Verification items for the finished model (mm, model axes). Face numbers are marked on the shaded views. A direction names the side the tool comes from. Round coordinates to 2 decimals unless told otherwise and drop trailing zeros. Write each loop counter-clockwise with the first axis right and the second up, starting at its lowest first coordinate (ties: lowest second). Pieces come first, ordered by that corner, then holes.
from build123d import *

# Parameters (mm, degrees)
SKETCH_1_R           = 7.505
SKETCH_1_R_2         = 2.505
EXTRUDE_1_DEPTH      = 10
EXTRUDE_3_DEPTH      = 18.25
EXTRUDE_3_DEPTH_BACK = 7
SKETCH_7_W           = 8
SKETCH_7_H           = 10
SKETCH_9_W           = 8
SKETCH_9_H           = 3.5
CUT_EXTRUDE_1_DEPTH  = 18.25
SKETCH_10_R          = 7.505
SKETCH_10_R_2        = 2.505
EXTRUDE_4_DEPTH      = 10
SKETCH_11_R          = 2.505
CUT_EXTRUDE_2_DEPTH  = 10


with BuildPart() as part:
    # 草圖1 → 伸長-薄件1 (new body)
    with BuildSketch(Plane(origin=(0, 0, 0), x_dir=(1, 0, 0), z_dir=(0, 1, 0))):
        Circle(SKETCH_1_R)
        Circle(SKETCH_1_R_2, mode=Mode.SUBTRACT)
    extrude(amount=EXTRUDE_1_DEPTH)

    # 草圖7 → 填料-伸長3 (add, two sides: drawn at the far end of the back side and taken through both)
    with BuildSketch(Plane.XY.offset(13).offset(-EXTRUDE_3_DEPTH_BACK)):
        with Locations((0, 5)):
            Rectangle(SKETCH_7_W, SKETCH_7_H)
    extrude(amount=EXTRUDE_3_DEPTH + EXTRUDE_3_DEPTH_BACK)

    # 草圖9 → 除料-伸長1 (cut)
    with BuildSketch(Plane(origin=(0, 10, 0), x_dir=(1, 0, 0), z_dir=(0, 1, 0))):
        with Locations((0, -29.5)):
            Rectangle(SKETCH_9_W, SKETCH_9_H)
    extrude(amount=-CUT_EXTRUDE_1_DEPTH, mode=Mode.SUBTRACT)

    # 草圖10 → 伸長-薄件4 (add)
    with BuildSketch(Plane(origin=(0, 10, 0), x_dir=(1, 0, 0), z_dir=(0, 1, 0))):
        with Locations((0, -27.75)):
            Circle(SKETCH_10_R)
        with Locations((0, -27.75)):
            Circle(SKETCH_10_R_2, mode=Mode.SUBTRACT)
    extrude(amount=-EXTRUDE_4_DEPTH)

    # 草圖11 → 除料-伸長2 (cut)
    with BuildSketch(Plane(origin=(0, 10, 0), x_dir=(1, 0, 0), z_dir=(0, 1, 0))):
        with Locations(Location((0, -27.75, 0), (0, 0, 270))):
            Circle(SKETCH_11_R)
    extrude(amount=-CUT_EXTRUDE_2_DEPTH, mode=Mode.SUBTRACT)


solid = part.part
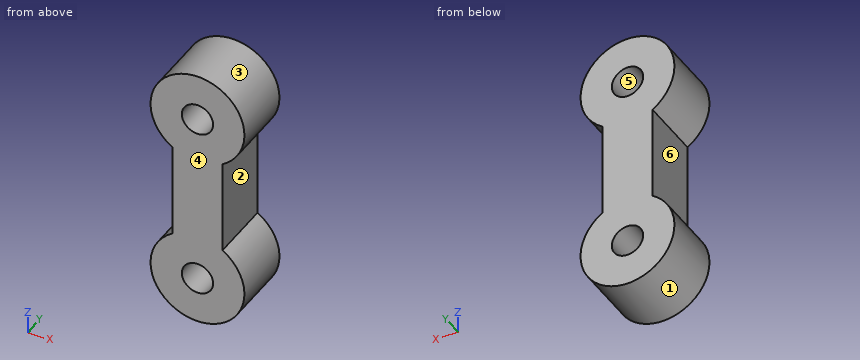
Q1. Depth check by flat-ended pin: P1, Ø5, axis at y = 5.5, z = 15.5, coming from the -X side; P2, Ø3, axis at x = 3, y = 4.5, coming from the -Z side; P3, Ø6, axis at y = 7.5, z = 9.5, coming from the +X side; P4, Ø4.5, axis at x = 0, z = 27.75, coming from the +Y side. Enter the tip coordinate at first touch or a pass-through.
Recorded:
P1: stops at x = -4
P2: stops at z = -7.35
P3: stops at x = 4
P4: passes through
Q2. Sectioned sample at B-B (z = 27.75). Enter the section's corners in (x, y) (3 decimals).
Recorded:
outline: (-7.505, 0) - (-2.505, 0) - (-2.505, 10) - (-7.505, 10) - close; (2.505, 0) - (7.505, 0) - (7.505, 10) - (2.505, 10) - close
Q3. Sectioned sample at D-D (y = 7). Enter the section's corners in (x, z) (3 decimals).
Recorded:
outline: (-4, 6.35) arc R7.505 ccw (long way) to (4, 6.35) - (4, 21.4) arc R7.505 ccw (long way) to (-4, 21.4) - close; hole circle Ø5.01 at (0, 0); hole circle Ø5.01 at (0, 27.75)
Q4. Release check for a two-part mould opening along X. For the marked faces 3, 4, 5 and 6 record: released by +X, released by -X, zero draft, split by the parting line, or undercut.
Recorded:
face 3: split by the parting line
face 4: zero draft
face 5: undercut
face 6: released by -X
Q5. Tool access check on the marked faces 1 and 2. Record the directions out of +Z, -Z, +X, -X, +Y, -Y that give a thin tool (end or side, any length) a straight path to the whole face; none if there is none.
Recorded:
face 1: +Y, -Y
face 2: +X, +Y, -Y
Q6. Material ranges on line 1 along Z through (x, y) = (0, 6.5) (3 decimals); line 2 along Z through (x, y) = (1.25, 3.25); line 3 along X through (y, z) = (2.5, 0) (3 decimals), recorded low to high.
Recorded:
line 1: z = -7.505 to -2.505, 2.505 to 25.245, 30.255 to 35.255
line 2: z = -7.4 to -2.17, 2.17 to 25.58, 29.92 to 35.15
line 3: x = -7.505 to -2.505, 2.505 to 7.505
Q7. Sectioned sample at A-A (x = 0). Enter the section's corners in (y, z) (3 decimals).
Recorded:
outline: (0, -7.505) - (10, -7.505) - (10, -2.505) - (0, -2.505) - close; (0, 2.505) - (10, 2.505) - (10, 25.245) - (0, 25.245) - close; (0, 30.255) - (10, 30.255) - (10, 35.255) - (0, 35.255) - close
Q8. Sectioned sample at C-C (x = -6). Enter the section's corners in (y, z), plus the area to 3 significant figures.
Recorded:
outline: (0, -4.51) - (10, -4.51) - (10, 4.51) - (0, 4.51) - close; (0, 23.24) - (10, 23.24) - (10, 32.26) - (0, 32.26) - close
area: 180 mm2
